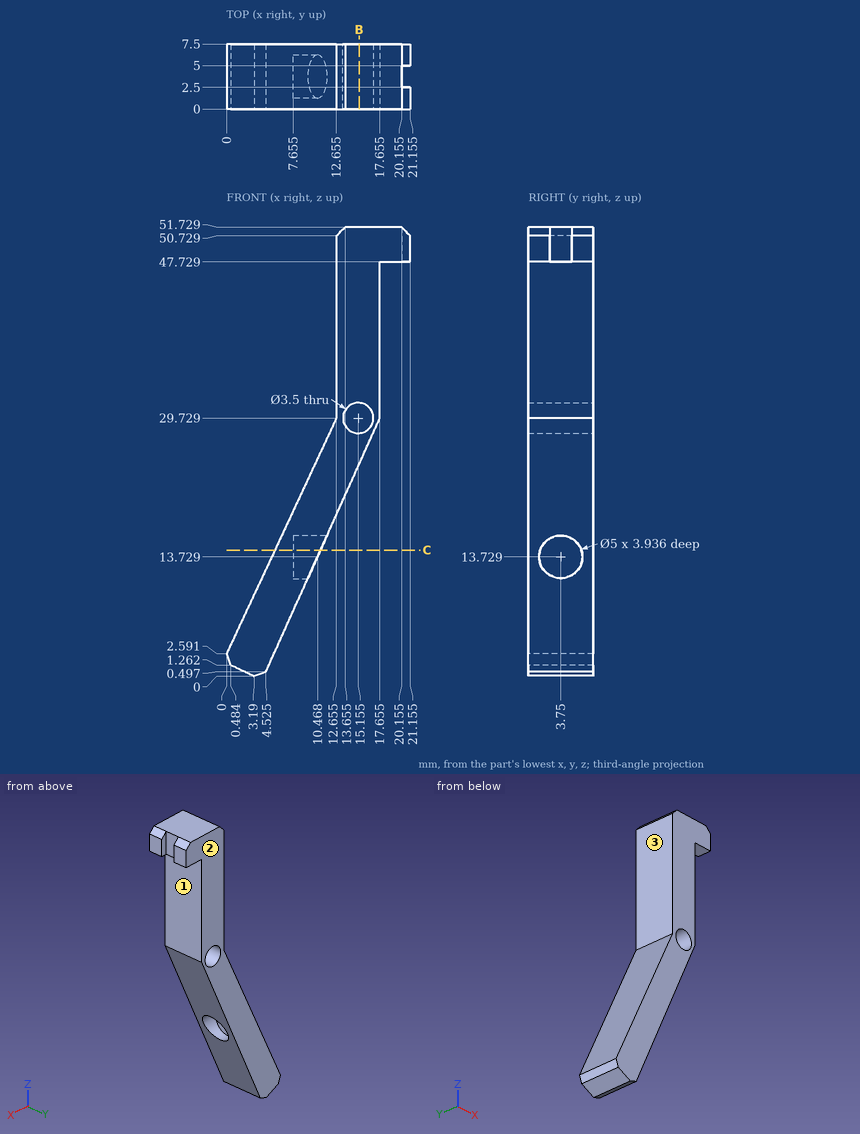
Study the drawing (mm; zero at the part's minimum x, y, z) and answer. A direction names the side the tool comes from. Give positions to 0.01 mm unless a question says otherwise; leave off trailing zeros. Loops run counter-clockwise (first coordinate to the right, second up) from the corner with the lowest first, then second, coordinate; pieces in that order, holes last. Notation, with made-up numbers: M -15,22.25 L 39,22.25 A18 ccw 39,50.25 Z; hole C 71,17 d5. An arc over 180 degrees is marked long. One line per item, written item: value. Start each with the question number.
1. Which of the six approach directions +Z, -Z, +X, -X, +Y, -Y give full straight-line access (tool end or side, diameter ignored) to the marked faces 1, 2 and 3?
2. Find section C-C (z = 14.5). Give the vertices of the cut face in (x, y) (1 decimal).
3. Each of these flat-tipped pins is pushed along its axis until it touches: P1, Ø1.5, axis at y = 5.5, z = 9.5, coming from the -X side; P2, Ø1.5, axis at x = 10.5, y = 4, coming from the +Z side (1 decimal); P3, Ø1.5, axis at x = 7, y = 6, coming from the +Z side. Where does it stop, or does it pass through?
4. Find the intervals of material crossed by probe 1 along X at (y, z) = (6, 36.5) (1 decimal); probe 2 along Z at (x, y) = (14, 5.5) (1 decimal); probe 3 along X at (y, z) = (5.75, 28.5) (1 decimal), in increasing order.
5. Find section B-B (x = 15.25). Give the vertices of the cut face in (y, z) (1 decimal), and give its area (3 significant figures).
Reported:
1. face 1: -Z, +X, +Y, -Y
1. face 2: +Z, -Z, +X, -X, +Y
1. face 3: +Z, -X, +Y, -Y
2. outline: M 5.6,0 L 10.8,0 L 10.8,1.4 L 7.7,1.4 L 7.7,6.1 L 10.8,6.1 L 10.8,7.5 L 5.6,7.5 Z
3. P1: stops at x = 2.87
3. P2: stops at z = 26.7
3. P3: stops at z = 19.21
4. probe 1: x = 12.7 to 17.7
4. probe 2: z = 21.6 to 28.4, 31 to 51.7
4. probe 3: x = 12.1 to 13.9, 16.4 to 17.1
5. outline: M 0,24.4 L 7.5,24.4 L 7.5,28 L 0,28 Z; M 0,31.5 L 7.5,31.5 L 7.5,51.7 L 0,51.7 Z
5. area: 179 mm²
